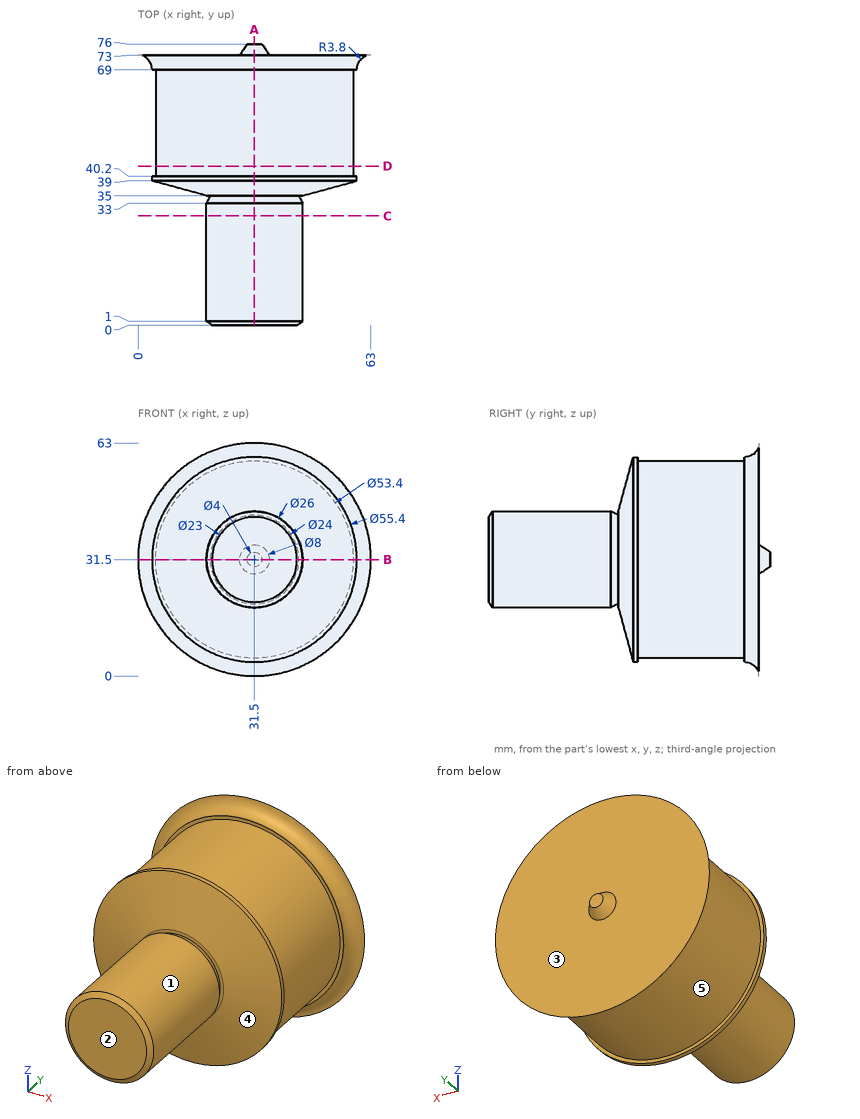
Could you check a few things on this drawing? It's one solid part, dimensions in mm from its lowest x, y, z. A direction names the side the tool comes from. Coordinates: 2 decimals unless noted, no trailing zeros. Order: outer loops, then holes, each group sorted by start corner. A loop starts at its lowest first (then second) coordinate and runs counter-clockwise, first axis right, second up. Notation, with made-up numbers: (-36, 50.5) - (14, 50.5) arc R26 cw to (14, 78.5) - close; hole circle Ø2 at (64.5, 79.5). An arc over 180 degrees is marked (long way). One line per question, with ' | ' between items. Start each with the question number.
1. If we section it at C-C (y = 29.5): Write out the boundary of the cut face in (x, z).
2. I'm going to push flat-ended pins straight in: pin 1 Ø3 at (x, z) = (15.5, 45.5) entering from +Y; pin 2 Ø2 at (x, y) = (29.5, 25) entering from -Z; pin 3 Ø2 at (x, y) = (54.5, 62.5) entering from -Z. Where does each tip first touch, or does it pass through?
3. If we section it at A-A (x = 31.5): Write out the boundary of the cut face in (y, z).
4. If we section it at D-D (y = 43): Write out the boundary of the cut face in (x, z).
5. Please list where these lines run through material, in increasing order: line 1 along Y through (x, z) = (39.5, 23.5); line 2 along Y through (x, z) = (28, 17); line 3 along X through (y, z) = (65.5, 38). Write a range as [from, to].
6. Which directions (+Z, -Z, +X, -X, +Y, -Y) give clear straight access to the entire face, cutting with the end or side of a thin tool? Please do the marked faces 1 and 2.
7. If we mould it in two halves opening along Y, with no side actions, what happens to the marked faces 3, 4 and 5? For each: released by +Y, released by -Y, zero draft, split by the parting line, or undercut.
8. If we section it at B-B (z = 31.5): Write out the boundary of the cut face in (x, y), and give its area (3 significant figures).
Model answer:
1) outline: circle Ø26 at (31.5, 31.5)
2) pin 1: stops at y = 73 | pin 2: stops at z = 18.54 | pin 3: stops at z = 16.37
3) outline: (0, 20) - (1, 18.5) - (33, 18.5) - (35, 19.5) - (35, 18.5) - (39, 3.8) - (40.2, 3.8) - (40.2, 4.8) - (69, 4.8) - (69, 3.8) - (69.2, 3.8) arc R3.8 cw to (73, 0) - (73, 27.5) - (76, 29.5) - (76, 33.5) - (73, 35.5) - (73, 63) arc R3.8 cw to (69.2, 59.2) - (69, 59.2) - (69, 58.2) - (40.2, 58.2) - (40.2, 59.2) - (39, 59.2) - (35, 44.5) - (35, 43.5) - (33, 44.5) - (1, 44.5) - (0, 43) - close
4) outline: circle Ø53.4 at (31.5, 31.5)
5) line 1: y = [0, 73] | line 2: y = [35.52, 73] | line 3: x = [5.6, 57.4]
6) face 1: -Y | face 2: +Z, -Z, +X, -X, -Y
7) face 3: released by +Y | face 4: released by -Y | face 5: undercut
8) outline: (0, 73) arc R3.8 cw to (3.8, 69.2) - (3.8, 69) - (4.8, 69) - (4.8, 40.2) - (3.8, 40.2) - (3.8, 39) - (18.5, 35) - (19.5, 35) - (18.5, 33) - (18.5, 1) - (20, 0) - (43, 0) - (44.5, 1) - (44.5, 33) - (43.5, 35) - (44.5, 35) - (59.2, 39) - (59.2, 40.2) - (58.2, 40.2) - (58.2, 69) - (59.2, 69) - (59.2, 69.2) arc R3.8 cw to (63, 73) - (35.5, 73) - (33.5, 76) - (29.5, 76) - (27.5, 73) - close | area: 2,920 mm²
